The listing builds one solid part. Answer for the finished solid, in the listing's coordinates (mm). A direction names the side the tool comes from. Round coordinates to 2 decimals unless told otherwise and drop trailing zeros. Loops run counter-clockwise (first coordinate to the right, second up) from the corner with the lowest first, then second, coordinate; pieces in that order, holes last. Notation, with made-up numbers: M 2.25,74.5 L 51.25,74.5 A18 cw 51.25,90.5 Z; hole C 21,51 d1. An arc over 180 degrees is marked long. Answer as a JSON object with one key per item and string values.
Autodesk Inventor part; units mm, degrees
ref_plane "YZ Plane" through (0, 0, 0) normal (1, 0, 0) x (0, 1, 0)
ref_plane "XZ Plane" through (0, 0, 0) normal (0, 1, 0) x (-1, 0, 0)
ref_plane "XY Plane" through (0, 0, 0) normal (0, 0, 1) x (1, 0, 0)
sketch "Sketch1" plane through (0, 0, 0) normal (0, 0, 1) x (1, 0, 0)
  line L0 (0, 17.9605) -> (17.9605, 0) construction
  line L1 (17.9605, 0) -> (0, -17.9605) construction
  line L2 (0, -17.9605) -> (-17.9605, 0) construction
  line L3 (-17.9605, 0) -> (0, 17.9605) construction
  line L4 (0, 17.9605) -> (0, -17.9605) construction
  line L5 (17.9605, 0) -> (-17.9605, 0) construction
  line L6 (0, 17.9605) -> (-17.9605, 0)
  line L7 (0, -86.3372) -> (0, 55.9028)
  line L8 (-58.674, 0) -> (58.674, 0)
  line L9 (0, 17.9605) -> (17.9605, 0)
  line L10 (17.9605, 0) -> (0, -17.9605)
  line L11 (-17.9605, 0) -> (0, -17.9605)
  line L12 (0, 25.1447) -> (-25.1447, 0)
  line L13 (-25.1447, 0) -> (0, -25.1447)
  line L14 (0, -25.1447) -> (25.1447, 0)
  line L15 (25.1447, 0) -> (0, 25.1447)
  line L16 (-41.91, 35.5828) -> (41.91, 35.5828)
  line L17 (41.91, 35.5828) -> (41.91, -66.0172)
  line L18 (41.91, -66.0172) -> (-41.91, -66.0172)
  line L19 (-41.91, -66.0172) -> (-41.91, 35.5828)
  point P0 (0, 0)
  point P1 (0, 0)
  point P2 (0, 0)
  point P3 (0, 0)
  point P4 (0, 0)
  point P5 (29.7157, 21.8287)
  point P6 (0, 35.5828)
  dimension "d0" = 25.4
  dimension "d1" = 25.4
  dimension "d5" = 0
  dimension "d6" = 5.08
  dimension "d7" = 5.08
  dimension "d15" = 83.82
  dimension "d16" = 101.6
extrude "Extrusion2" add sketch "Sketch1" along normal blind 20.32 contours L6 L8 L12 L7 | L7 L15 L8 L9 | L11 L7 L13 L8 | L8 L14 L7 L10
extrude "Extrusion3" add sketch "Sketch1" along normal blind 12.7 contours L12 L8 L19 L16 L7 | L7 L16 L17 L8 L15 | L13 L7 L18 L19 L8 | L8 L17 L18 L7 L14
sketch "Sketch2" plane through (41.91, -66.0172, 0) normal (1, 0, 0) x (0, 0, -1)
  line L0 (0, 0) -> (0, 101.6)
  line L1 (0, 101.6) -> (-12.7, 101.6)
  line L2 (-12.7, 0) -> (-12.7, 101.6)
  line L3 (0, 0) -> (-12.7, 0)
  line L4 (-42.9388, 0) -> (30.2388, 0)
  line L5 (30.2388, 0) -> (30.2388, 9.2066)
  line L6 (30.2388, 9.2066) -> (-42.9388, 9.2066)
  line L7 (-42.9388, 9.2066) -> (-42.9388, 0)
  line L8 (-42.9388, 0) -> (30.2388, 9.2066) construction
  line L9 (30.2388, 0) -> (-42.9388, 9.2066) construction
  point P0 (0, 66.0172)
  point P1 (-6.35, 4.6033)
  point P2 (-6.35, 0)
extrude "Extrusion4" add sketch "Sketch2" against normal up to surface (83.82 mm away) contours L3 L2 L6 L0 | L0 L6 L5 L4 | L4 L7 L6 L2
equation "\"d7\" = d6"
properties part number "base_end_mounts" material "ABS Plastic"
Item 1: Determine the mould class of faces 1 (the face through (-10, -10, 0)), 2 (the face through (12.396, -12.748, 16.457)), 3 (the face through (-8.85, 9.11, 10.02)), 4 (the face through (1, -66.017, 6)) for opening direction Y: released by +Y, released by -Y, zero draft, split by the parting line, or undercut.
Values follow:
{"face 1": "zero draft", "face 2": "undercut", "face 3": "undercut", "face 4": "released by -Y"}
Item 2: The part is cut by section D-D (y = 11). Give the vertices of the cut face in (x, z), then the cut area to 3 significant figures.
Values follow:
{"outline": "M -41.91,0 L -6.96,0 L -6.96,20.32 L -14.14,20.32 L -14.14,12.7 L -41.91,12.7 Z; M 6.96,0 L 41.91,0 L 41.91,12.7 L 14.14,12.7 L 14.14,20.32 L 6.96,20.32 Z", "area": "997 mm^2"}
Item 3: Straight lines are drawn through the part: line 1 (Y direction, x = 1.5, z = 15); line 2 (Y direction, x = -1.5, z = 24.5); line 3 (X direction, y = 6, z = 13.5). For each, find the intervals that lie inside material, in ascending order.
Values follow:
{"line 1": "-66.02 to -56.81, -23.64 to -16.46, 16.46 to 23.64", "line 2": "-66.02 to -56.81", "line 3": "-19.14 to -11.96, 11.96 to 19.14"}
Item 4: The part is cut by section C-C (z = 10). Give the vertices of the cut face in (x, y), then the cut area to 3 significant figures.
Values follow:
{"outline": "M -41.91,-66.02 L 41.91,-66.02 L 41.91,35.58 L -41.91,35.58 Z; hole M -17.96,0 L 0,-17.96 L 17.96,0 L 0,17.96 Z", "area": "7,870 mm^2"}
Item 5: Which of the six approach directions +Z, -Z, +X, -X, +Y, -Y give full straight-line access (tool end or side, diameter ignored) to faces 5 (the face through (-12.748, -12.396, 16.457)), 6 (the face through (-9.4, -9.2, 20.32)), 7 (the face through (1, -56.811, -15)), 8 (the face through (8.85, 9.11, 10.02)), 9 (the face through (1, -56.811, 28))?
Values follow:
{"face 5": "+Z, -X", "face 6": "+Z, +X, -X, +Y", "face 7": "-Z, +X, -X, +Y", "face 8": "+Z, -Z", "face 9": "+Z, +X, -X"}
Item 6: Flat-ended cylindrical pins translate along their axes: P1, Ø15, axis at x = -3, y = -10.5, coming from the +Z side; P2, Ø5, axis at x = 22.5, z = -16, coming from the +Y side; P3, Ø8, axis at x = -27.5, y = -45.5, coming from the -Z side; P4, Ø10, axis at y = -48.5, z = 34.5, coming from the -X side. Find the tip coordinate at first contact, or state that the pin passes through.
Values follow:
{"P1": "z = 20.32", "P2": "y = -56.81", "P3": "z = 0", "P4": "through"}
Item 7: The part is cut by section B-B (x = 2). Give the vertices of the cut face in (y, z).
Values follow:
{"outline": "M -66.02,-30.24 L -56.81,-30.24 L -56.81,0 L -15.96,0 L -15.96,20.32 L -23.14,20.32 L -23.14,12.7 L -56.81,12.7 L -56.81,42.94 L -66.02,42.94 Z; M 15.96,0 L 35.58,0 L 35.58,12.7 L 23.14,12.7 L 23.14,20.32 L 15.96,20.32 Z"}
Item 8: The part is cut by section A-A (z = 19). Give the vertices of the cut face in (x, y).
Values follow:
{"outline": "M -41.91,-66.02 L 41.91,-66.02 L 41.91,-56.81 L -41.91,-56.81 Z; M -25.14,0 L 0,-25.14 L 25.14,0 L 0,25.14 Z; hole M -17.96,0 L 0,-17.96 L 17.96,0 L 0,17.96 Z"}
